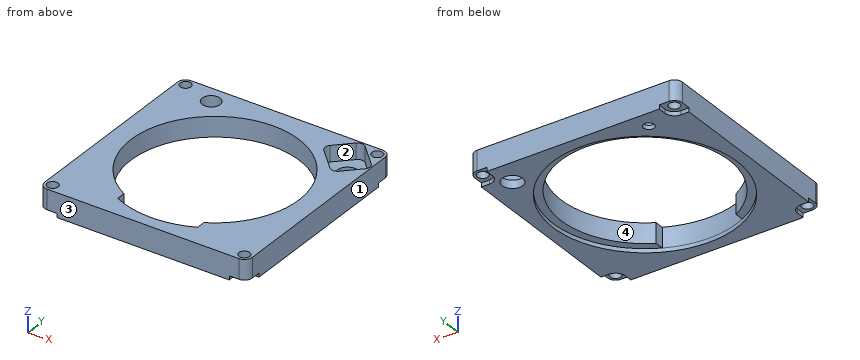
from build123d import *

# Parameters (mm, degrees)
BOSS_EXTRUDE1_DEPTH      = 7.9375
SKETCH2_R                = 36.5125
BOSS_EXTRUDE2_DEPTH      = 1.5875
F_6_CLEARANCE_HOLE1_D    = 4.3053
SKETCH5_R                = 3.57124
CUT_EXTRUDE1_DEPTH       = 7.9375
CUT_EXTRUDE2_REACH       = 3.588
SKETCH6_R                = 2.1
CUT_EXTRUDE3_DEPTH       = 6.35
F_5_16_CLEARANCE_HOLE1_D = 8.2042


with BuildPart() as part:
    # Sketch1 → Boss-Extrude1 (new body)
    with BuildSketch(Plane.XY):
        with BuildLine():
            Line((-38.1, -41.275), (38.1, -41.275))
            ThreePointArc((38.1, -41.275), (40.34506403, -40.34506403), (41.275, -38.1))
            Line((41.275, -38.1), (41.275, 38.1))
            ThreePointArc((41.275, 38.1), (40.34506403, 40.34506403), (38.1, 41.275))
            Line((38.1, 41.275), (-38.1, 41.275))
            ThreePointArc((-38.1, 41.275), (-40.34506403, 40.34506403), (-41.275, 38.1))
            Line((-41.275, 38.1), (-41.275, -38.1))
            ThreePointArc((-41.275, -38.1), (-40.34506403, -40.34506403), (-38.1, -41.275))
        make_face()
        with BuildLine():
            Line((15.875, -29.315069184), (15.875, -32.880800344))
            ThreePointArc((15.875, -32.880800344), (0, -36.5125), (-15.875, -32.880800344))
            Line((-15.875, -32.880800344), (-15.875, -29.315069184))
            ThreePointArc((-15.875, -29.315069184), (0, 33.3375), (15.875, -29.315069184))
        make_face(mode=Mode.SUBTRACT)
    extrude(amount=-BOSS_EXTRUDE1_DEPTH)

    # Sketch2 → Boss-Extrude2 (add)
    with BuildSketch(Plane(origin=(0, 0, -7.9375), x_dir=(-1, 0, 0), z_dir=(0, 0, -1))):
        with BuildLine():
            Line((-34.290000001, -38.1), (-34.290000001, -41.275))
            Line((-34.290000001, -41.275), (34.289999999, -41.275))
            Line((34.289999999, -41.275), (34.289999999, -38.1))
            ThreePointArc((34.289999999, -38.1), (35.405923163, -35.405923164), (38.099999999, -34.29))
            Line((38.099999999, -34.29), (41.274999999, -34.29))
            Line((41.274999999, -34.29), (41.274999999, 34.29))
            Line((41.274999999, 34.29), (38.099999999, 34.29))
            ThreePointArc((38.099999999, 34.29), (35.405923163, 35.405923164), (34.289999999, 38.1))
            Line((34.289999999, 38.1), (34.289999999, 41.275))
            Line((34.289999999, 41.275), (-34.290000001, 41.275))
            Line((-34.290000001, 41.275), (-34.290000001, 38.1))
            ThreePointArc((-34.290000001, 38.1), (-35.405923165, 35.405923164), (-38.100000001, 34.29))
            Line((-38.100000001, 34.29), (-41.275000001, 34.29))
            Line((-41.275000001, 34.29), (-41.275000001, -34.29))
            Line((-41.275000001, -34.29), (-38.100000001, -34.29))
            ThreePointArc((-38.100000001, -34.29), (-35.405923165, -35.405923164), (-34.290000001, -38.1))
        make_face()
        Circle(SKETCH2_R, mode=Mode.SUBTRACT)
    extrude(amount=BOSS_EXTRUDE2_DEPTH)

    # #6 Clearance Hole1 (through all)
    with Locations(Plane(origin=(0, 0, -7.9375), x_dir=(-1, 0, 0), z_dir=(0, 0, -1))):
        with Locations((-38.1, 38.1), (38.099999999, 38.1), (38.1, -38.1), (-38.1, -38.1)):
            Hole(F_6_CLEARANCE_HOLE1_D / 2)

    # Sketch5 → Cut-Extrude1 (cut)
    with BuildSketch(Plane.XY):
        with Locations((-25.4, 34.417)):
            Circle(SKETCH5_R)
    extrude(amount=-CUT_EXTRUDE1_DEPTH, mode=Mode.SUBTRACT)

    # Sketch6 → Cut-Extrude2 (cut, up to next)
    with BuildSketch(Plane.XY.offset(-7.9375), mode=Mode.PRIVATE) as cut_extrude2_sk1:
        with Locations((-25.4, 34.417)):
            Circle(SKETCH6_R)
    cut_extrude2_tool1 = extrude(cut_extrude2_sk1.sketch, amount=-CUT_EXTRUDE2_REACH, mode=Mode.PRIVATE) & part.part
    add(cut_extrude2_tool1.solids().sort_by_distance((-25.4, 34.417, -7.9375))[0], mode=Mode.SUBTRACT)

    # Sketch7 → Cut-Extrude3 (cut)
    with BuildSketch(Plane.XY):
        with BuildLine():
            Line((22.254952032, 30.270714503), (30.270714503, 22.254952032))
            ThreePointArc((30.270714503, 22.254952032), (32.066765727, 21.511003256), (33.862816952, 22.254952032))
            Line((33.862816952, 22.254952032), (39.975047968, 28.367183048))
            ThreePointArc((39.975047968, 28.367183048), (40.718996744, 30.163234273), (39.975047968, 31.959285497))
            Line((39.975047968, 31.959285497), (31.959285497, 39.975047968))
            ThreePointArc((31.959285497, 39.975047968), (30.163234273, 40.718996744), (28.367183048, 39.975047968))
            Line((28.367183048, 39.975047968), (22.254952032, 33.862816952))
            ThreePointArc((22.254952032, 33.862816952), (21.511003256, 32.066765727), (22.254952032, 30.270714503))
        make_face()
    extrude(amount=-CUT_EXTRUDE3_DEPTH, mode=Mode.SUBTRACT)

    # 5/16 Clearance Hole1 (through all)
    with Locations(Plane(origin=(0, 0, -9.525), x_dir=(-1, 0, 0), z_dir=(0, 0, -1))):
        with Locations((-31.115, 31.115)):
            Hole(F_5_16_CLEARANCE_HOLE1_D / 2)


solid = part.part
For this review, take the finished solid that the model builds, in its own axes (mm). Face numbers are marked on the shaded views. Coordinates: 2 decimals unless noted, no trailing zeros. Loops run counter-clockwise (first coordinate to the right, second up) from the corner with the lowest first, then second, coordinate; pieces in that order, holes last. Notation, with made-up numbers: (-10.5, 31.5) - (48.5, 31.5) arc R27 cw to (48.5, 55.5) - close; hole circle Ø7 at (-39, 32). An arc over 180 degrees is marked (long way). Return JSON: item names as keys, results as strings.
Item 1: Take a section at A-A (x = 0). Give the boundary of the cut face in (y, z) (1 decimal), then the cut area to 3 significant figures.
Determined:
{"outline": "(-41.3, -9.5) - (-36.5, -9.5) - (-36.5, 0) - (-41.3, 0) - close; (33.3, -7.9) - (36.5, -7.9) - (36.5, -9.5) - (41.3, -9.5) - (41.3, 0) - (33.3, 0) - close", "area": "116 mm2"}
Item 2: For line 1 (Y direction, x = -38.1, z = -2.5) (3 decimals); line 2 (Y direction, x = 0, z = -6) (1 decimal); line 3 (Y direction, x = 38.1, z = -3.75) (3 decimals), list the stretches that pass through material, from the lowest coordinate up.
Determined:
{"line 1": "y = -41.275 to -40.253, -35.947 to 35.947, 40.253 to 41.275", "line 2": "y = -41.3 to -36.5, 33.3 to 41.3", "line 3": "y = -41.275 to -40.253, -35.947 to 26.492, 33.834 to 35.947, 40.253 to 41.275"}
Item 3: Take a section at D-D (x = -25.4). Give the boundary of the cut face in (y, z) (1 decimal).
Determined:
{"outline": "(-41.3, -9.5) - (-26.2, -9.5) - (-26.2, -7.9) - (-21.6, -7.9) - (-21.6, 0) - (-41.3, 0) - close; (21.6, -7.9) - (26.2, -7.9) - (26.2, -9.5) - (32.3, -9.5) - (32.3, -7.9) - (30.8, -7.9) - (30.8, 0) - (21.6, 0) - close; (36.5, -9.5) - (41.3, -9.5) - (41.3, 0) - (38, 0) - (38, -7.9) - (36.5, -7.9) - close"}
Item 4: Take a section at C-C (z = -3). State how many separate pieces and enclosed holes the cut face has, then the cut area to 3 significant figures.
Determined:
{"separate pieces": "1", "enclosed holes": "7", "area": "2,890 mm2"}
Item 5: Take a section at B-B (y = -15). Give the boundary of the cut face in (x, z) (1 decimal).
Determined:
{"outline": "(-41.3, -9.5) - (-33.3, -9.5) - (-33.3, -7.9) - (-29.8, -7.9) - (-29.8, 0) - (-41.3, 0) - close; (29.8, -7.9) - (33.3, -7.9) - (33.3, -9.5) - (41.3, -9.5) - (41.3, 0) - (29.8, 0) - close"}
Item 6: Mouldability with a two-part tool opening along Y and no side actions: class the marked faces 1, 2, 3 and 4 as pulls with the +Y half, pulls with the -Y half, needs draft (parallel to the pull), parting line crosses it, or undercut.
Determined:
{"face 1": "needs draft", "face 2": "undercut", "face 3": "pulls with the -Y half", "face 4": "undercut"}
Item 7: Insertion check: pin 1 (0.8 mm diameter, centred on x = 40, z = -8.5, fed in from +Y); pin 2 (5.5 mm diameter, centred on x = -37.5, y = 38.5, fed in from -Z); pin 3 (0.8 mm diameter, centred on y = 40.5, z = -8.5, fed in from -X). Each pin has a flat end and moves straight along its axis. Give the tip position at first contact, or say it passes through.
Determined:
{"pin 1": "stops at y = 34.29", "pin 2": "stops at z = -7.94", "pin 3": "stops at x = -34.29"}
